from build123d import *

# Parameters (mm, degrees)
SKETCH27_R                  = 5
SKETCH27_R_2                = 2.5
BOSS_EXTRUDE1_DEPTH         = 8
TAP_DRILL_FOR_M3_TAP1_D     = 2.5
TAP_DRILL_FOR_M3_TAP1_DEPTH = 10
TAP_DRILL_FOR_M3_TAP1_TIP   = 0.751075774
SKETCH33_R                  = 7.99
CUT_EXTRUDE2_DEPTH          = 5


with BuildPart() as part:
    # Sketch27 → Boss-Extrude1 (new body)
    with BuildSketch(Plane(origin=(0, 0, 0), x_dir=(0, 0, -1), z_dir=(1, 0, 0))):
        with BuildLine():
            Line((12, 48), (37.349351573, 48))
            Line((37.349351573, 48), (37.349351573, 25))
            Line((37.349351573, 25), (35.981694484, 7.531672014))
            ThreePointArc((35.981694484, 7.531672014), (31.842856312, 2.290019211), (25.420672816, 4.12317623))
            Line((25.420672816, 4.12317623), (3.604566829, 29.892489756))
            ThreePointArc((3.604566829, 29.892489756), (2.020455604, 41.626952956), (12, 48))
        make_face()
        with Locations((12, 37)):
            Circle(SKETCH27_R, mode=Mode.SUBTRACT)
        with Locations((30, 8)):
            Circle(SKETCH27_R_2, mode=Mode.SUBTRACT)
    extrude(amount=BOSS_EXTRUDE1_DEPTH)

    # Tap Drill for M3 Tap1
    with Locations(Plane(origin=(0, 0, -37.349351573), x_dir=(-1, 0, 0), z_dir=(0, 0, -1))):
        with Locations((-3, 32), (-3, 44)):
            Hole(TAP_DRILL_FOR_M3_TAP1_D / 2, depth=TAP_DRILL_FOR_M3_TAP1_DEPTH)
            with Locations((0, 0, -(TAP_DRILL_FOR_M3_TAP1_DEPTH + TAP_DRILL_FOR_M3_TAP1_TIP / 2))):  # 118° drill point
                Cone(0, TAP_DRILL_FOR_M3_TAP1_D / 2, TAP_DRILL_FOR_M3_TAP1_TIP, mode=Mode.SUBTRACT)

    # Sketch33 → Cut-Extrude2 (cut)
    with BuildSketch(Plane(origin=(8, 0, 0), x_dir=(0, 0, -1), z_dir=(1, 0, 0))):
        with Locations((12, 37)):
            Circle(SKETCH33_R)
    extrude(amount=-CUT_EXTRUDE2_DEPTH, mode=Mode.SUBTRACT)


solid = part.part
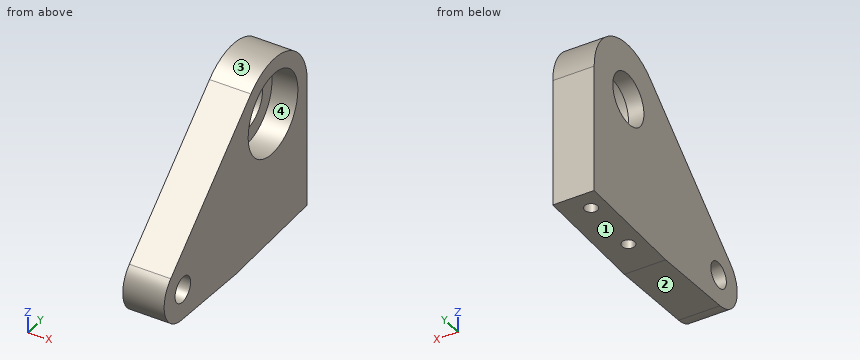
Read the model definition and answer for the solid it produces. Units are mm, in the model's axes. Face numbers are marked on the shaded views. Give positions to 0.01 mm unless a question says otherwise; leave off trailing zeros. Write each loop counter-clockwise with the first axis right and the second up, starting at its lowest first coordinate (ties: lowest second). Pieces come first, ordered by that corner, then holes. Notation, with made-up numbers: (-31, 67) - (0, 67) arc R5 ccw to (0, 75) - close; hole circle Ø8 at (19, -39.75). An arc over 180 degrees is marked (long way). Use CSV: the item, a comma, the result in double quotes. Start each with the question number.
Item 1: The part is cut by section C-C, the plane y = 39. Give the vertices of the cut face in (x, z).
Item 2: The part is cut by section A-A, the plane z = -29. Give the vertices of the cut face in (x, y), and give its area (3 significant figures).
Item 3: The part is cut by section B-B, the plane x = 1. Give the vertices of the cut face in (y, z), and give its area (3 significant figures).
Item 4: The mould has two halves that part along Y. Classify the marked faces 1, 2, 3 and 4: pulls with the +Y half, pulls with the -Y half, needs draft (parallel to the pull), parting line crosses it, or undercut.
Item 5: Consider line 1 (Z direction, x = 1.15, y = 37); line 2 (X direction, y = 44, z = -32); line 3 (Y direction, x = 4, z = -30). Determine where each line is inside the solid, lowest interval first.
Item 6: The part is cut by section D-D, the plane z = -11. Give the vertices of the cut face in (x, y), and give its area (3 significant figures).
Item 7: Flat-ended cylindrical pins translate along their axes: P1, Ø8, axis at y = 8, z = -30, coming from the -X side; P2, Ø4, axis at x = 1.5, y = 16.5, coming from the +Z side. Find the tip coordinate at first contact, or state that the pin passes through.
Taken from the geometry:
1,outline,"(0, -37.35) - (8, -37.35) - (8, -19.74) - (3, -19.74) - (3, -16.58) - (0, -16.58) - close; (0, -7.42) - (3, -7.42) - (3, -4.26) - (8, -4.26) - (8, -1.18) - (0, -1.18) - close"
2,outline,"(0, 2.08) - (8, 2.08) - (8, 5.71) - (0, 5.71) - close; (0, 10.29) - (8, 10.29) - (8, 48) - (0, 48) - close; hole circle Ø2.5 at (3, 32); hole circle Ø2.5 at (3, 44)"
2,area,"321 mm2"
3,outline,"(4.12, -25.42) arc R6 ccw to (7.53, -35.98) - (25, -37.35) - (48, -37.35) - (48, -12) arc R11 ccw to (29.89, -3.6) - close; hole circle Ø5 at (8, -30); hole circle Ø10 at (37, -12)"
3,area,"1,110 mm2"
4,face 1,"needs draft"
4,face 2,"pulls with the -Y half"
4,face 3,"parting line crosses it"
4,face 4,"undercut"
5,line 1,"-37.35 to -17, -7 to -1"
5,line 2,"0 to 1.75, 4.25 to 8"
5,line 3,"2 to 5.5, 10.5 to 31.25, 32.75 to 43.25, 44.75 to 48"
6,outline,"(0, 21.16) - (8, 21.16) - (8, 29.07) - (3, 29.07) - (3, 32.1) - (0, 32.1) - close; (0, 41.9) - (3, 41.9) - (3, 44.93) - (8, 44.93) - (8, 47.95) - (0, 47.95) - close"
6,area,"106 mm2"
7,P1,"x = 0"
7,P2,"z = -13.25"
